```python
from build123d import *

# Parameters (mm, degrees)
SKETCH_1_R          = 6
EXTRUDE_1_DEPTH     = 6
SKETCH_1_4_R        = 3
CUT_EXTRUDE_2_DEPTH = 3
HOLE_WIZARD_M3_1_D  = 3.2


with BuildPart() as part:
    # ｽｹｯﾁ1 → ﾎﾞｽ - 押し出し1 (new body)
    with BuildSketch(Plane.XY):
        Circle(SKETCH_1_R)
    extrude(amount=-EXTRUDE_1_DEPTH)

    # ｽｹｯﾁ1<4> → ｶｯﾄ - 押し出し2 (cut)
    with BuildSketch(Plane.XY):
        Circle(SKETCH_1_4_R)
    extrude(amount=-CUT_EXTRUDE_2_DEPTH, mode=Mode.SUBTRACT)

    # M3 すきま穴1 (through all)
    with Locations(Plane(origin=(0, 0, -6), x_dir=(-1, 0, 0), z_dir=(0, 0, -1))):
        with Locations((0, 0)):
            Hole(HOLE_WIZARD_M3_1_D / 2)


solid = part.part
```
Design review of the part built by this model. Coordinates are the model's own, in mm. Give positions to 0.01 mm unless a question says otherwise; leave off trailing zeros. Write each loop counter-clockwise with the first axis right and the second up, starting at its lowest first coordinate (ties: lowest second). Pieces come first, ordered by that corner, then holes.
(1) Mouldability with a two-part tool opening along Y and no side actions: class faces 1 (the face through (-3, -1, 0)), 2 (the face through (-3, 0, -1)), 3 (the face through (1.3, -1.3, -3)), 4 (the face through (-6, 0, -3)) as +Y half, -Y half, draft (parallel to the pull), parting line (faces both ways), or undercut.
Checked values:
face 1: draft
face 2: undercut
face 3: undercut
face 4: parting line
(2) Add section C-C (z = -4.7). Give the boundary of the cut face in (x, y), and give its area (3 significant figures).
Checked values:
outline: circle Ø12 at (0, 0); hole circle Ø3.2 at (0, 0)
area: 105 mm2
(3) Add section D-D (y = 2.5). Give the boundary of the cut face in (x, z), and give its area (3 significant figures).
Checked values:
outline: (-5.45, -6) - (5.45, -6) - (5.45, 0) - (1.66, 0) - (1.66, -3) - (-1.66, -3) - (-1.66, 0) - (-5.45, 0) - close
area: 55.5 mm2
(4) Wall thickness on line 1 along Y through (x, z) = (0, -0.95); line 2 along Y through (x, z) = (0, -4.2); line 3 along X through (y, z) = (-2.75, -2.05): over which ranges is each line inside the solid? List them lowest first.
Checked values:
line 1: y = -6 to -3, 3 to 6
line 2: y = -6 to -1.6, 1.6 to 6
line 3: x = -5.33 to -1.2, 1.2 to 5.33
(5) Clearance check with flat-ended pins moving along their axes: pin 1 Ø5 at (x, y) = (0, 0) entering from +Z; pin 2 Ø1.5 at (x, z) = (2, -3) entering from -Y; pin 3 Ø1 at (x, z) = (-2.5, -4) entering from -Y. State where each tip first meets the part, or that it passes through.
Checked values:
pin 1: stops at z = -3
pin 2: stops at y = -5.87
pin 3: stops at y = -5.66
(6) Add section A-A (y = 0). Give the boundary of the cut face in (x, z).
Checked values:
outline: (-6, -6) - (-1.6, -6) - (-1.6, -3) - (-3, -3) - (-3, 0) - (-6, 0) - close; (1.6, -6) - (6, -6) - (6, 0) - (3, 0) - (3, -3) - (1.6, -3) - close
